from build123d import *

# Parameters (mm, degrees)
F1_DEPTH = 30
F4_DEPTH = 27.7
F7_DEPTH = 50.2


with BuildPart() as f1:
    # F0 (on Top) → F1 (new body)
    with BuildSketch(Plane.XY):
        Polygon((-1.3985362389, 20), (0, 0), (172, 0), (173.3985362389, 20), align=None)
    extrude(amount=F1_DEPTH)

    # F3 (on face) → F4 (cut, symmetric)
    with BuildSketch(Plane(origin=(0, 0, 0), x_dir=(-0.9975640503, -0.0697564737, 0), z_dir=(-0.0697564737, 0.9975640503, 0))):
        Polygon((-2.4909883108, 35.6227924818), (0, 0), (0, 35.6227924818), align=None)
    extrude(amount=F4_DEPTH, both=True, mode=Mode.SUBTRACT)

    # F6 (on face) → F7 (cut, symmetric)
    with BuildSketch(Plane(origin=(0.8369460882, 11.9688866826, 0), x_dir=(-0.9975640503, 0.0697564737, 0), z_dir=(0.0697564737, 0.9975640503, 0))):
        Polygon((-171.5810166447, 89.9730579068), (-171.5810166447, 0), (-165.3201019088, 89.5352520994), align=None)
    extrude(amount=F7_DEPTH, both=True, mode=Mode.SUBTRACT)


solid = f1.part
Could you check a few things on this model? Use its own coordinates, in mm. Coordinates: 2 decimals unless noted, no trailing zeros. Order: outer loops, then holes, each group sorted by start corner. A loop starts at its lowest first (then second) coordinate and runs counter-clockwise, first axis right, second up. Notation, with made-up numbers: (35.25, 37.25) - (78.25, 37.25) arc R32 cw to (78.25, 66.25) - close; hole circle Ø3 at (29.25, 81.5). An arc over 180 degrees is marked (long way). Answer in a Markdown table with one row per item. Add a question column.
(1) If we section it at B-B, the plane y = 12: Please give me the cut outline in (x, z), then the cut area to 3 significant figures.
(2) I need wall thicknesses on L1, parallel to X at y = 6.5, z = 6; L2, parallel to X at y = 3.25, z = 13. Which ranges of each line are inside material? Lowest first, please.
(3) Will these pins go through, and if not, where does the flat tip stop? pin 1 (4 mm diameter, centred on y = 15, z = 4, fed in from -X); pin 2 (3 mm diameter, centred on y = 2.5, z = 6.5, fed in from -X); pin 3 (6 mm diameter, centred on y = 17, z = 11.5, fed in from -X); pin 4 (5 mm diameter, centred on x = 23.5, z = 14.5, fed in from -Y).
(4) If we section it at A-A, the plane z = 12.5: Please give me the cut outline in (x, y).
Results are:
| question | item | result |
|---|---|---|
| 1 | outline | (-0.84, 0) - (172.84, 0) - (170.74, 30) - (1.26, 30) - close |
| 1 | area | 5,150 mm2 |
| 2 | L1 | x = -0.03 to 172.03 |
| 2 | L2 | x = 0.68 to 171.32 |
| 3 | pin 1 | stops at x = -0.97 |
| 3 | pin 2 | stops at x = 0.13 |
| 3 | pin 3 | stops at x = -0.68 |
| 3 | pin 4 | stops at y = 0 |
| 4 | outline | (-0.52, 20) - (0.88, 0) - (171.12, 0) - (172.52, 20) - close |
